Autodesk Inventor part; units mm, degrees
ref_plane "Arbeitsebene1" through (34.1, -565, 450) normal (0, 1, 0) x (0, 0, 1)
ref_plane "YZ Plane" through (0, 0, 0) normal (1, 0, 0) x (0, 1, 0)
ref_plane "XZ Plane" through (0, 0, 0) normal (0, 1, 0) x (-1, 0, 0)
sketch "Skizze1" plane through (0, 0, 0) normal (0, 0, 1) x (1, 0, 0)
  line L0 (0, 0) -> (32, 0) construction
  line L1 (-84, 5) -> (-84, -35)
  line L2 (-84, -35) -> (116, -35)
  line L3 (116, -35) -> (116, 5)
  line L4 (-84, 5) -> (116, 5)
  line L5 (0, 0) -> (-84, 0) construction
  line L6 (32, 0) -> (116, 0) construction
  point P0 (16, 5)
  dimension "d0" = 200
  dimension "d1" = 40
  dimension "d2" = 5
extrude "Extrusion1" add sketch "Skizze1" along normal blind 40
sketch "Skizze2" plane through (0, 0, 40) normal (0, 0, 1) x (1, 0, 0)
  line L0 (116, -35) -> (116, 5)
  line L1 (-84, 5) -> (-84, -35)
  line L2 (116, -35) -> (76, -35)
  line L3 (76, -35) -> (76, 5)
  line L4 (76, 5) -> (116, 5)
  line L5 (-84, -35) -> (-44, -35)
  line L6 (-44, -35) -> (-44, 5)
  line L7 (-44, 5) -> (-84, 5)
  point P0 (0, 0)
extrude "Extrusion2" add sketch "Skizze2" along normal blind 475
sketch "Skizze3" plane through (0, 0, 515) normal (0, 0, 1) x (1, 0, 0)
  line L0 (116, -35) -> (116, 5)
  line L1 (-84, 5) -> (-84, -35)
  line L2 (76, -35) -> (116, -35)
  line L3 (116, -35) -> (-84, -35)
  line L4 (116, 5) -> (-84, 5)
  point P0 (0, 0)
extrude "Extrusion3" add sketch "Skizze3" against normal blind 40
ref_plane "Arbeitsebene1" through (34.1, -565, 450) normal (0, 1, 0) x (0, 0, 1)
sketch "Skizze4" plane through (-84, -35, 0) normal (0, -1, 0) x (1, 0, 0)
  line L0 (136.45, -16.1) -> (139.75, -16.1) construction
  line L1 (138.1, -16.1) -> (138.1, 515) construction
  line L2 (0, 515) -> (200, 515) construction
  line L3 (160, 515) -> (200, 515)
  line L4 (200, 515) -> (200, 475)
  line L5 (200, 475) -> (160, 475)
  line L6 (160, 475) -> (160, 515)
  line L7 (200, 0) -> (200, 515)
  point P0 (84, 0)
  dimension "d10" = 40
  dimension "d26" = 40
  dimension "d27" = 0
extrude "Extrusion4" add sketch "Skizze4" along normal blind 500
equation "\"d5\" = höheFrame"
properties part number "FrameSide" material "Aluminium 6061, Frame"
Input: part model. Units: mm. Frame: model coordinates. A direction names the side the tool comes from. Coordinates: 2 decimals unless noted, no trailing zeros. Write each loop counter-clockwise with the first axis right and the second up, starting at its lowest first coordinate (ties: lowest second). Pieces come first, ordered by that corner, then holes. Notation, with made-up numbers: (65.5, 36) - (73.5, 36) arc R20 ccw to (73.5, 42) - close; hole circle Ø1 at (54.25, 13.5). An arc over 180 degrees is marked (long way). Put each result on its own line as item: value. Start each with the question number.
1) Cut plane D-D (x = -66). Return the cut outline in (y, z).
2) Cut plane A-A (x = 10.5). Return the cut outline in (y, z), plus the area to 3 significant figures.
3) Contact query for flat-ended pins moving along their axis: pin 1 (20 mm diameter, centred on x = 88, y = -178.5, fed in from -Z); pin 2 (12 mm diameter, centred on y = -270.5, z = 497, fed in from -X); pin 3 (12 mm diameter, centred on x = 13.5, y = -8, fed in from -Z). Output: stop coordinate, or through.
4) Reachability of faces 5 (the face through (15, -15, 40)), 6 (the face through (116, -144, 488)), 7 (the face through (76, -282, 495)) from +Z, -Z, +X, -X, +Y, -Y: full face, straight path, thin tool, end or side. Return the list, or none.
5) Cut plane C-C (y = -322). Return the cut outline in (x, z).
6) Mould query, pull axis Z, two halves, no side actions, for faces 1 (the face through (96, -535, 495)), 2 (the face through (15, -15, 475)), 3 (the face through (96, -282, 475)), 4 (the face through (82, -204, 515)). Classes: pulls with the +Z half, pulls with the -Z half, needs draft (parallel to the pull), parting line crosses it, or undercut.
7) Ray query, L1, parallel to Y at x = -74.5, z = 37.5; L2, parallel to Z at x = 107.5, y = -280.5. Return the intervals inside material, ascending.
8) Cut plane B-B (z = 314.5). Return the cut outline in (x, y), plus the area to 3 significant figures.
Resolved:
1. outline: (-35, 0) - (5, 0) - (5, 515) - (-35, 515) - close
2. outline: (-35, 0) - (5, 0) - (5, 40) - (-35, 40) - close; (-35, 475) - (5, 475) - (5, 515) - (-35, 515) - close
2. area: 3,200 mm2
3. pin 1: stops at z = 475
3. pin 2: stops at x = 76
3. pin 3: stops at z = 0
4. face 5: +Y, -Y
4. face 6: +Z, -Z, +X, +Y, -Y
4. face 7: +Z, -Z, -X, -Y
5. outline: (76, 475) - (116, 475) - (116, 515) - (76, 515) - close
6. face 1: needs draft
6. face 2: undercut
6. face 3: pulls with the -Z half
6. face 4: pulls with the +Z half
7. L1: y = -35 to 5
7. L2: z = 475 to 515
8. outline: (-84, -35) - (-44, -35) - (-44, 5) - (-84, 5) - close; (76, -35) - (116, -35) - (116, 5) - (76, 5) - close
8. area: 3,200 mm2
